Study the drawing (mm; zero at the part's minimum x, y, z) and answer. A direction names the side the tool comes from. Coordinates: 2 decimals unless noted, no trailing zeros. Loops run counter-clockwise (first coordinate to the right, second up) from the corner with the lowest first, then second, coordinate; pieces in that order, holes last. Notation, with made-up numbers: (37.5, -37) - (96.5, -37) arc R25 ccw to (96.5, 1) - close; hole circle Ø9 at (77.5, 63). An arc over 180 degrees is marked (long way). Write each question's results on one line, items separated by ' | '. Start each with the question number.
(1) For the marked faces 1 and 2, determine the directions among +Z, -Z, +X, -X, +Y, -Y from which every point of the face is accessible in a straight line to the end or side of a thin tool.
(2) Find section A-A on z = 7. Determine the outline of the cut face in (x, y), then the cut area to 3 significant figures.
(3) Consider line 1 (Y direction, x = 50.5, z = 11); line 2 (Z direction, x = 23, y = 2.75) (1 decimal); line 3 (X direction, y = 5.5, z = 10) (1 decimal). Determine where each line is inside the solid, lowest interval first. Write a range as from..to.
(4) Determine the mould class of the marked faces 3, 4 and 5 for opening direction X: released by +X, released by -X, zero draft, split by the parting line, or undercut.
(5) Given pin 1 Ø10 at (y, z) = (4.5, 12) entering from +X; pin 2 Ø1.5 at (y, z) = (6.5, 34.5) entering from +X; pin 3 Ø3 at (x, z) = (47.5, 37.5) entering from -Y, each flat-ended and moving along its own axis, determine where each tip first touches the part or whether it passes through.
(6) Find section C-C on x = 23. Determine the outline of the cut face in (y, z), then the cut area to 3 significant figures.
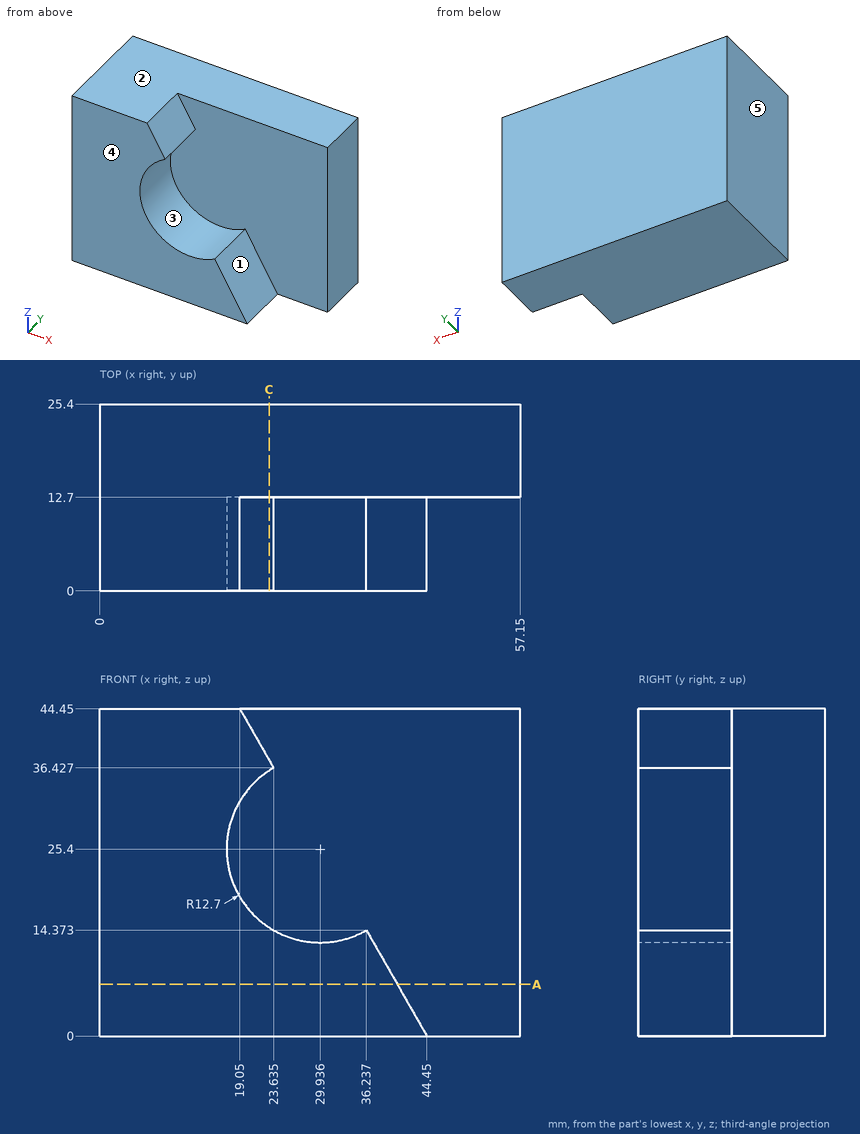
Values:
1) face 1: +Z, +X, -Y | face 2: +Z, +X, -X, +Y, -Y
2) outline: (0, 0) - (40.45, 0) - (40.45, 12.7) - (57.15, 12.7) - (57.15, 25.4) - (0, 25.4) - close | area: 1,240 mm²
3) line 1: y = 12.7..25.4 | line 2: z = 0..14.8, 36..37.5 | line 3: x = 0..38.7
4) face 3: undercut | face 4: zero draft | face 5: released by -X
5) pin 1: stops at x = 40.45 | pin 2: stops at x = 21.92 | pin 3: stops at y = 12.7
6) outline: (0, 0) - (25.4, 0) - (25.4, 44.45) - (12.7, 44.45) - (12.7, 37.54) - (0, 37.54) - (0, 36.04) - (12.7, 36.04) - (12.7, 14.76) - (0, 14.76) - close | area: 771 mm²
